Model file for the job. Use its own axes, mm. A direction names the side the tool comes from. Round coordinates to 2 decimals unless told otherwise and drop trailing zeros. Order: outer loops, then holes, each group sorted by start corner. A loop starts at its lowest first (then second) coordinate and runs counter-clockwise, first axis right, second up. Notation, with made-up numbers: M 24.25,50 L 40.25,50 A19 ccw 40.25,59 Z; hole C 17.25,-19.75 d7. An arc over 180 degrees is marked long. Return JSON: item names as keys, results as strings. Group by question number.
Item 1: Pin check, flat tips, straight feed: pin 1 Ø3 at (x, y) = (25.4, 940.816) entering from +Z; pin 2 Ø7 at (x, y) = (25.4, 581.152) entering from -Z (3 decimals). Stop position of each tip, or through.
Item 2: Probe line 1 along X through (y, z) = (494, -19.5) (3 decimals); line 2 along X through (y, z) = (401.32, -1.65); line 3 along Z through (x, y) = (9, 1044) (3 decimals). List the from-to ranges inside material, lowest first.
Item 3: Slice it at C-C on x = 15. Write the cut outline in (y, z) (3 decimals), then the cut area to 3 significant figures.
Item 4: Which spindle directions (+Z, -Z, +X, -X, +Y, -Y) get a long thin tool onto all of the face, cutting with end or side? Do faces 1 (the face through (27, 0, -2)), 2 (the face through (3.175, 576, -14)). Say none if no direction does.
Item 5: Pull direction X, two halves, no side cores. Call faces 3 (the face through (26, 576, -3.175)), 4 (the face through (27, 1168.4, -2)), 5 (the face through (0, 576, -13)), 6 (the face through (50.8, 576, -13)): pulls with the +X half, pulls with the -X half, needs draft (parallel to the pull), parting line crosses it, or undercut.
Item 6: Slice it at A-A on z = -7. Write the cut outline in (x, y) (3 decimals), then the cut area to 3 significant figures.
Item 7: Slice it at B-B on y = 1084.5. Write the cut outline in (x, z) (3 decimals).
from build123d import *

# Parameters (mm, degrees)
BOSS_EXTRUDE1_DEPTH = 1168.4
CUT_EXTRUDE1_REACH  = 27.4
SKETCH2_R           = 2.667
CUT_EXTRUDE2_REACH  = 27.4
SKETCH4_R           = 1.5875


with BuildPart() as part:
    # Sketch1 → Boss-Extrude1 (new body)
    with BuildSketch(Plane(origin=(0, 0, 0), x_dir=(1, 0, 0), z_dir=(0, 1, 0))):
        Polygon((3.175, 3.175), (3.175, 25.4), (0, 25.4), (0, 0), (50.8, 0), (50.8, 25.4), (47.625, 25.4), (47.625, 3.175), align=None)
    extrude(amount=BOSS_EXTRUDE1_DEPTH)

    # Sketch2 → Cut-Extrude1 (cut, up to next)
    with BuildSketch(Plane.XY, mode=Mode.PRIVATE) as cut_extrude1_sk1:
        with Locations((25.4, 101.6)):
            Circle(SKETCH2_R)
    cut_extrude1_tool1 = extrude(cut_extrude1_sk1.sketch, amount=-CUT_EXTRUDE1_REACH, mode=Mode.PRIVATE) & part.part
    add(cut_extrude1_tool1.solids().sort_by_distance((25.4, 101.6, 0))[0], mode=Mode.SUBTRACT)
    # Sketch2 → Cut-Extrude1 (cut, up to next)
    with BuildSketch(Plane.XY, mode=Mode.PRIVATE) as cut_extrude1_sk2:
        with Locations((25.4, 161.544)):
            Circle(SKETCH2_R)
    cut_extrude1_tool2 = extrude(cut_extrude1_sk2.sketch, amount=-CUT_EXTRUDE1_REACH, mode=Mode.PRIVATE) & part.part
    add(cut_extrude1_tool2.solids().sort_by_distance((25.4, 161.544, 0))[0], mode=Mode.SUBTRACT)
    # Sketch2 → Cut-Extrude1 (cut, up to next)
    with BuildSketch(Plane.XY, mode=Mode.PRIVATE) as cut_extrude1_sk3:
        with Locations((25.4, 221.488)):
            Circle(SKETCH2_R)
    cut_extrude1_tool3 = extrude(cut_extrude1_sk3.sketch, amount=-CUT_EXTRUDE1_REACH, mode=Mode.PRIVATE) & part.part
    add(cut_extrude1_tool3.solids().sort_by_distance((25.4, 221.488, 0))[0], mode=Mode.SUBTRACT)
    # Sketch2 → Cut-Extrude1 (cut, up to next)
    with BuildSketch(Plane.XY, mode=Mode.PRIVATE) as cut_extrude1_sk4:
        with Locations((25.4, 281.432)):
            Circle(SKETCH2_R)
    cut_extrude1_tool4 = extrude(cut_extrude1_sk4.sketch, amount=-CUT_EXTRUDE1_REACH, mode=Mode.PRIVATE) & part.part
    add(cut_extrude1_tool4.solids().sort_by_distance((25.4, 281.432, 0))[0], mode=Mode.SUBTRACT)
    # Sketch2 → Cut-Extrude1 (cut, up to next)
    with BuildSketch(Plane.XY, mode=Mode.PRIVATE) as cut_extrude1_sk5:
        with Locations((25.4, 341.376)):
            Circle(SKETCH2_R)
    cut_extrude1_tool5 = extrude(cut_extrude1_sk5.sketch, amount=-CUT_EXTRUDE1_REACH, mode=Mode.PRIVATE) & part.part
    add(cut_extrude1_tool5.solids().sort_by_distance((25.4, 341.376, 0))[0], mode=Mode.SUBTRACT)
    # Sketch2 → Cut-Extrude1 (cut, up to next)
    with BuildSketch(Plane.XY, mode=Mode.PRIVATE) as cut_extrude1_sk6:
        with Locations((25.4, 401.32)):
            Circle(SKETCH2_R)
    cut_extrude1_tool6 = extrude(cut_extrude1_sk6.sketch, amount=-CUT_EXTRUDE1_REACH, mode=Mode.PRIVATE) & part.part
    add(cut_extrude1_tool6.solids().sort_by_distance((25.4, 401.32, 0))[0], mode=Mode.SUBTRACT)
    # Sketch2 → Cut-Extrude1 (cut, up to next)
    with BuildSketch(Plane.XY, mode=Mode.PRIVATE) as cut_extrude1_sk7:
        with Locations((25.4, 461.264)):
            Circle(SKETCH2_R)
    cut_extrude1_tool7 = extrude(cut_extrude1_sk7.sketch, amount=-CUT_EXTRUDE1_REACH, mode=Mode.PRIVATE) & part.part
    add(cut_extrude1_tool7.solids().sort_by_distance((25.4, 461.264, 0))[0], mode=Mode.SUBTRACT)
    # Sketch2 → Cut-Extrude1 (cut, up to next)
    with BuildSketch(Plane.XY, mode=Mode.PRIVATE) as cut_extrude1_sk8:
        with Locations((25.4, 521.208)):
            Circle(SKETCH2_R)
    cut_extrude1_tool8 = extrude(cut_extrude1_sk8.sketch, amount=-CUT_EXTRUDE1_REACH, mode=Mode.PRIVATE) & part.part
    add(cut_extrude1_tool8.solids().sort_by_distance((25.4, 521.208, 0))[0], mode=Mode.SUBTRACT)
    # Sketch2 → Cut-Extrude1 (cut, up to next)
    with BuildSketch(Plane.XY, mode=Mode.PRIVATE) as cut_extrude1_sk9:
        with Locations((25.4, 581.152)):
            Circle(SKETCH2_R)
    cut_extrude1_tool9 = extrude(cut_extrude1_sk9.sketch, amount=-CUT_EXTRUDE1_REACH, mode=Mode.PRIVATE) & part.part
    add(cut_extrude1_tool9.solids().sort_by_distance((25.4, 581.152, 0))[0], mode=Mode.SUBTRACT)
    # Sketch2 → Cut-Extrude1 (cut, up to next)
    with BuildSketch(Plane.XY, mode=Mode.PRIVATE) as cut_extrude1_sk10:
        with Locations((25.4, 641.096)):
            Circle(SKETCH2_R)
    cut_extrude1_tool10 = extrude(cut_extrude1_sk10.sketch, amount=-CUT_EXTRUDE1_REACH, mode=Mode.PRIVATE) & part.part
    add(cut_extrude1_tool10.solids().sort_by_distance((25.4, 641.096, 0))[0], mode=Mode.SUBTRACT)
    # Sketch2 → Cut-Extrude1 (cut, up to next)
    with BuildSketch(Plane.XY, mode=Mode.PRIVATE) as cut_extrude1_sk11:
        with Locations((25.4, 701.04)):
            Circle(SKETCH2_R)
    cut_extrude1_tool11 = extrude(cut_extrude1_sk11.sketch, amount=-CUT_EXTRUDE1_REACH, mode=Mode.PRIVATE) & part.part
    add(cut_extrude1_tool11.solids().sort_by_distance((25.4, 701.04, 0))[0], mode=Mode.SUBTRACT)
    # Sketch2 → Cut-Extrude1 (cut, up to next)
    with BuildSketch(Plane.XY, mode=Mode.PRIVATE) as cut_extrude1_sk12:
        with Locations((25.4, 760.984)):
            Circle(SKETCH2_R)
    cut_extrude1_tool12 = extrude(cut_extrude1_sk12.sketch, amount=-CUT_EXTRUDE1_REACH, mode=Mode.PRIVATE) & part.part
    add(cut_extrude1_tool12.solids().sort_by_distance((25.4, 760.984, 0))[0], mode=Mode.SUBTRACT)
    # Sketch2 → Cut-Extrude1 (cut, up to next)
    with BuildSketch(Plane.XY, mode=Mode.PRIVATE) as cut_extrude1_sk13:
        with Locations((25.4, 820.928)):
            Circle(SKETCH2_R)
    cut_extrude1_tool13 = extrude(cut_extrude1_sk13.sketch, amount=-CUT_EXTRUDE1_REACH, mode=Mode.PRIVATE) & part.part
    add(cut_extrude1_tool13.solids().sort_by_distance((25.4, 820.928, 0))[0], mode=Mode.SUBTRACT)
    # Sketch2 → Cut-Extrude1 (cut, up to next)
    with BuildSketch(Plane.XY, mode=Mode.PRIVATE) as cut_extrude1_sk14:
        with Locations((25.4, 880.872)):
            Circle(SKETCH2_R)
    cut_extrude1_tool14 = extrude(cut_extrude1_sk14.sketch, amount=-CUT_EXTRUDE1_REACH, mode=Mode.PRIVATE) & part.part
    add(cut_extrude1_tool14.solids().sort_by_distance((25.4, 880.872, 0))[0], mode=Mode.SUBTRACT)
    # Sketch2 → Cut-Extrude1 (cut, up to next)
    with BuildSketch(Plane.XY, mode=Mode.PRIVATE) as cut_extrude1_sk15:
        with Locations((25.4, 940.816)):
            Circle(SKETCH2_R)
    cut_extrude1_tool15 = extrude(cut_extrude1_sk15.sketch, amount=-CUT_EXTRUDE1_REACH, mode=Mode.PRIVATE) & part.part
    add(cut_extrude1_tool15.solids().sort_by_distance((25.4, 940.816, 0))[0], mode=Mode.SUBTRACT)
    # Sketch2 → Cut-Extrude1 (cut, up to next)
    with BuildSketch(Plane.XY, mode=Mode.PRIVATE) as cut_extrude1_sk16:
        with Locations((25.4, 1000.76)):
            Circle(SKETCH2_R)
    cut_extrude1_tool16 = extrude(cut_extrude1_sk16.sketch, amount=-CUT_EXTRUDE1_REACH, mode=Mode.PRIVATE) & part.part
    add(cut_extrude1_tool16.solids().sort_by_distance((25.4, 1000.76, 0))[0], mode=Mode.SUBTRACT)
    # Sketch2 → Cut-Extrude1 (cut, up to next)
    with BuildSketch(Plane.XY, mode=Mode.PRIVATE) as cut_extrude1_sk17:
        with Locations((25.4, 1060.704)):
            Circle(SKETCH2_R)
    cut_extrude1_tool17 = extrude(cut_extrude1_sk17.sketch, amount=-CUT_EXTRUDE1_REACH, mode=Mode.PRIVATE) & part.part
    add(cut_extrude1_tool17.solids().sort_by_distance((25.4, 1060.704, 0))[0], mode=Mode.SUBTRACT)
    # Sketch2 → Cut-Extrude1 (cut, up to next)
    with BuildSketch(Plane.XY, mode=Mode.PRIVATE) as cut_extrude1_sk18:
        with Locations((25.4, 1120.648)):
            Circle(SKETCH2_R)
    cut_extrude1_tool18 = extrude(cut_extrude1_sk18.sketch, amount=-CUT_EXTRUDE1_REACH, mode=Mode.PRIVATE) & part.part
    add(cut_extrude1_tool18.solids().sort_by_distance((25.4, 1120.648, 0))[0], mode=Mode.SUBTRACT)

    # Sketch4 → Cut-Extrude2 (cut, up to next)
    with BuildSketch(Plane.XY, mode=Mode.PRIVATE) as cut_extrude2_sk1:
        with Locations((25.4, 41.275)):
            Circle(SKETCH4_R)
    cut_extrude2_tool1 = extrude(cut_extrude2_sk1.sketch, amount=-CUT_EXTRUDE2_REACH, mode=Mode.PRIVATE) & part.part
    add(cut_extrude2_tool1.solids().sort_by_distance((25.4, 41.275, 0))[0], mode=Mode.SUBTRACT)
    # Sketch4 → Cut-Extrude2 (cut, up to next)
    with BuildSketch(Plane.XY, mode=Mode.PRIVATE) as cut_extrude2_sk2:
        with Locations((25.4, 12.7)):
            Circle(SKETCH4_R)
    cut_extrude2_tool2 = extrude(cut_extrude2_sk2.sketch, amount=-CUT_EXTRUDE2_REACH, mode=Mode.PRIVATE) & part.part
    add(cut_extrude2_tool2.solids().sort_by_distance((25.4, 12.7, 0))[0], mode=Mode.SUBTRACT)


solid = part.part
Output values:
{
 "1": {"pin 1": "through", "pin 2": "z = -3.175"},
 "2": {"line 1": "0 to 3.175, 47.625 to 50.8", "line 2": "0 to 22.73, 28.07 to 50.8", "line 3": "-3.175 to 0"},
 "3": {"outline": "M 0,-3.175 L 1168.4,-3.175 L 1168.4,0 L 0,0 Z", "area": "3,710 mm²"},
 "4": {"face 1": "+Z, -Z, +X, -X, -Y", "face 2": "-Z, +Y, -Y"},
 "5": {"face 3": "undercut", "face 4": "needs draft", "face 5": "pulls with the -X half", "face 6": "pulls with the +X half"},
 "6": {"outline": "M 0,0 L 3.175,0 L 3.175,1168.4 L 0,1168.4 Z; M 47.625,0 L 50.8,0 L 50.8,1168.4 L 47.625,1168.4 Z", "area": "7,420 mm²"},
 "7": {"outline": "M 0,-25.4 L 3.175,-25.4 L 3.175,-3.175 L 47.625,-3.175 L 47.625,-25.4 L 50.8,-25.4 L 50.8,0 L 0,0 Z"}
}
